```python
from build123d import *

# Parameters (mm, degrees)
SKETCH5_R          = 1.5
CUT_EXTRUDE1_DEPTH = 43.24020689


with BuildPart() as part:
    # Sketch4 → Revolve1 (revolve)
    with BuildSketch(Plane.XY, mode=Mode.PRIVATE) as revolve1_sk:
        Polygon((-8.5, 0), (-29.39375, 0), (-29.39375, -3), (-11.75, -3), (-11.75, -7.5), (-8.5, -7.5), align=None)
    revolve(revolve1_sk.sketch.rotate(Axis((0, 27.279243053, 0), (0, -1, 0)), 270), axis=Axis((0, 27.279243053, 0), (0, -1, 0)))

    # Sketch5 → Cut-Extrude1 (cut, through all)
    with BuildSketch(Plane(origin=(0, 0, 0), x_dir=(1, 0, 0), z_dir=(0, 1, 0))):
        with Locations(Location((-25, 0, 0), (0, 0, 270))):
            Circle(SKETCH5_R)
        with Locations(Location((-12.5, 21.650635095, 0), (0, 0, 270))):
            Circle(SKETCH5_R)
        with Locations(Location((12.5, 21.650635095, 0), (0, 0, 270))):
            Circle(SKETCH5_R)
        with Locations(Location((25, 0, 0), (0, 0, 270))):
            Circle(SKETCH5_R)
        with Locations(Location((12.5, -21.650635095, 0), (0, 0, 270))):
            Circle(SKETCH5_R)
        with Locations(Location((-12.5, -21.650635095, 0), (0, 0, 270))):
            Circle(SKETCH5_R)
    extrude(amount=-CUT_EXTRUDE1_DEPTH, mode=Mode.SUBTRACT)


solid = part.part
```
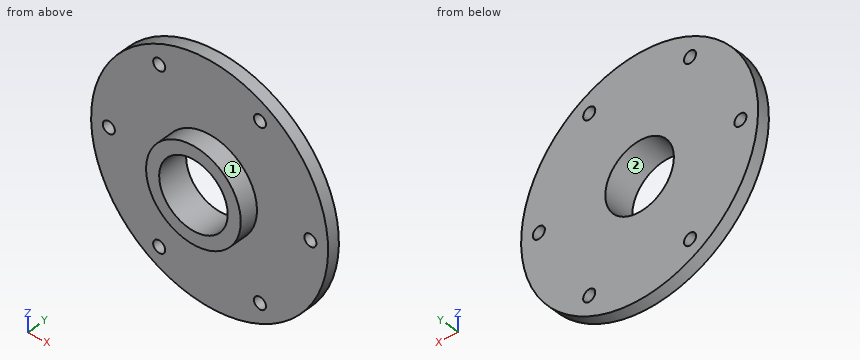
The model under review builds one solid part; all positions refer to its coordinate system, in mm. Face numbers are marked on the shaded views. A direction names the side the tool comes from. Coordinates: 2 decimals unless noted, no trailing zeros. Write each loop counter-clockwise with the first axis right and the second up, starting at its lowest first coordinate (ties: lowest second). Pieces come first, ordered by that corner, then holes.
1) We need section A-A on x = 0. State the section outline as (y, z) points.
2) To check wall thickness, follow probe 1 along X at (y, z) = (-0.65, 0); probe 2 along Y at (x, z) = (-16, 10); probe 3 along X at (y, z) = (-6.5, 2). State the ranges of each line that lie inside material, in increasing order.
3) Machinability: for the marked faces 1 and 2, which of the approach directions +Z, -Z, +X, -X, +Y, -Y give a long, thin tool a straight path to every point of the face, cutting with its end or side? Answer none if there is none.
4) We need section C-C on y = -1.25. State the section outline as (x, z) points, then the cut area to 3 significant figures.
5) We need section D-D on x = -12.5. State the section outline as (y, z) points.
6) We need section B-B on z = 0. State the section outline as (x, y) points, then the cut area to 3 significant figures.
7) Clearance check with flat-ended pins moving along their axes: pin 1 Ø3.5 at (x, z) = (25, 0) entering from -Y; pin 2 Ø2.5 at (x, z) = (12.5, -21.65) entering from -Y. State where each tip first meets the part, or that it passes through.
Answer list:
1. outline: (-7.5, -11.75) - (-3, -11.75) - (-3, -29.39) - (0, -29.39) - (0, -8.5) - (-7.5, -8.5) - close; (-7.5, 8.5) - (0, 8.5) - (0, 29.39) - (-3, 29.39) - (-3, 11.75) - (-7.5, 11.75) - close
2. probe 1: x = -29.39 to -26.5, -23.5 to -8.5, 8.5 to 23.5, 26.5 to 29.39
2. probe 2: y = -3 to 0
2. probe 3: x = -11.58 to -8.26, 8.26 to 11.58
3. face 1: -Y
3. face 2: +Y, -Y
4. outline: circle Ø58.79 at (0, 0); hole circle Ø3 at (-25, 0); hole circle Ø3 at (-12.5, -21.65); hole circle Ø3 at (-12.5, 21.65); hole circle Ø17 at (0, 0); hole circle Ø3 at (12.5, -21.65); hole circle Ø3 at (12.5, 21.65); hole circle Ø3 at (25, 0)
4. area: 2,440 mm2
5. outline: (-3, -26.6) - (0, -26.6) - (0, -23.15) - (-3, -23.15) - close; (-3, -20.15) - (0, -20.15) - (0, 20.15) - (-3, 20.15) - close; (-3, 23.15) - (0, 23.15) - (0, 26.6) - (-3, 26.6) - close
6. outline: (-29.39, -3) - (-26.5, -3) - (-26.5, 0) - (-29.39, 0) - close; (-23.5, -3) - (-11.75, -3) - (-11.75, -7.5) - (-8.5, -7.5) - (-8.5, 0) - (-23.5, 0) - close; (8.5, -7.5) - (11.75, -7.5) - (11.75, -3) - (23.5, -3) - (23.5, 0) - (8.5, 0) - close; (26.5, -3) - (29.39, -3) - (29.39, 0) - (26.5, 0) - close
6. area: 137 mm2
7. pin 1: stops at y = -3
7. pin 2: passes through
